```python
from build123d import *

# Parameters (mm, degrees)
SKETCH1_R           = 0.7
BOSS_EXTRUDE1_DEPTH = 0.8


with BuildPart() as part:
    # Sketch1 → Boss-Extrude1 (new body)
    with BuildSketch(Plane(origin=(0, 0, 0), x_dir=(0, 0, -1), z_dir=(1, 0, 0))):
        with BuildLine():
            ThreePointArc((3.228042319, 12.609235821), (1.223335432, 10.725526511), (3.968101377, 10.542577405))
            ThreePointArc((3.968101377, 10.542577405), (0.135522118, -0.982979757), (-3.697057141, 10.542577405))
            ThreePointArc((-3.697057141, 10.542577405), (-0.952291196, 10.725526511), (-2.956998083, 12.609235821))
            ThreePointArc((-2.956998083, 12.609235821), (0.135522118, -2.4118779), (3.228042319, 12.609235821))
        make_face()
        with Locations((2.635522118, 11.231222828)):
            Circle(SKETCH1_R, mode=Mode.SUBTRACT)
        with Locations(Location((-2.364477882, 11.231222828, 0), (0, 0, 180))):
            Circle(SKETCH1_R, mode=Mode.SUBTRACT)
    extrude(amount=BOSS_EXTRUDE1_DEPTH)


solid = part.part
```
Work out the finished part from the listing and answer in its coordinate system (mm). Round coordinates to 2 decimals unless told otherwise and drop trailing zeros. Write each loop counter-clockwise with the first axis right and the second up, starting at its lowest first coordinate (ties: lowest second). Pieces come first, ordered by that corner, then holes. Notation, with made-up numbers: (25.5, 18) -> (79.5, 18) arc R9 cw to (79.5, 31) -> close; hole circle Ø4 at (46.5, 47.5). An arc over 180 degrees is marked (long way). Write each question's results on one line, items separated by ' | '.
Q1. Section C-C, the plane y = 4.5 is taken. Write down the section's boundary in (x, z).
Data:
outline: (0, -7.91) -> (0.8, -7.91) -> (0.8, -6.47) -> (0, -6.47) -> close; (0, 6.2) -> (0.8, 6.2) -> (0.8, 7.64) -> (0, 7.64) -> close
Q2. Straight lines are drawn through the part: line 1 along Y through (x, z) = (0.6, 2.25); line 2 along Z through (x, y) = (0.55, 11); line 3 along Z through (x, y) = (0.3, 11.5). For each, find the intervals that lie inside material, in ascending order. Write a range as [from, to].
Data:
line 1: [-2.04, -0.52], [9.74, 10.54], [11.92, 12.73] | line 2: [-5.62, -3.3], [-1.97, -1.15], [0.88, 1.7], [3.03, 5.35] | line 3: [-5.06, -3.28], [-1.99, -1.16], [0.89, 1.72], [3.01, 4.79]
Q3. Flat-ended cylindrical pins translate along their axes: P1, Ø2, axis at y = 9, z = -2.5, coming from the -X side; P2, Ø1.5, axis at y = 2, z = -3, coming from the +X side. Find the tip coordinate at first contact, or state that the pin passes through.
Data:
P1: x = 0 | P2: through
Q4. Determine the mould class of faces 1 (the cylindrical face through (0.394, -2.406, 0.164)), 2 (the flat face through (0.8, 10.2, -2.4)), 3 (the cylindrical face through (0.39, 10.55, -2.48)) for opening direction Y: released by +Y, released by -Y, zero draft, split by the parting line, or undercut.
Data:
face 1: split by the parting line | face 2: zero draft | face 3: undercut
Q5. Section D-D, the plane x = 0.5 is taken. Write down the section's boundary in (y, z).
Data:
outline: (10.54, -3.97) arc R6.4 cw (long way) to (10.54, 3.7) arc R1.5 ccw (long way) to (12.61, 2.96) arc R7.83 ccw (long way) to (12.61, -3.23) arc R1.5 ccw (long way) to start; hole circle Ø1.4 at (11.23, -2.64); hole circle Ø1.4 at (11.23, 2.36)
Q6. Section B-B, the plane y = 11.5 is taken. Write down the section's boundary in (x, z), then the cut area to 3 significant figures.
Data:
outline: (0, -5.06) -> (0.8, -5.06) -> (0.8, -3.28) -> (0, -3.28) -> close; (0, -1.99) -> (0.8, -1.99) -> (0.8, -1.16) -> (0, -1.16) -> close; (0, 0.89) -> (0.8, 0.89) -> (0.8, 1.72) -> (0, 1.72) -> close; (0, 3.01) -> (0.8, 3.01) -> (0.8, 4.79) -> (0, 4.79) -> close | area: 4.18 mm^2
Q7. Section A-A, the plane z = 6 is taken. Write down the section's boundary in (x, y), then the cut area to 3 significant figures.
Data:
outline: (0, 0.55) -> (0.8, 0.55) -> (0.8, 3.6) -> (0, 3.6) -> close; (0, 7.24) -> (0.8, 7.24) -> (0.8, 10.28) -> (0, 10.28) -> close | area: 4.87 mm^2
